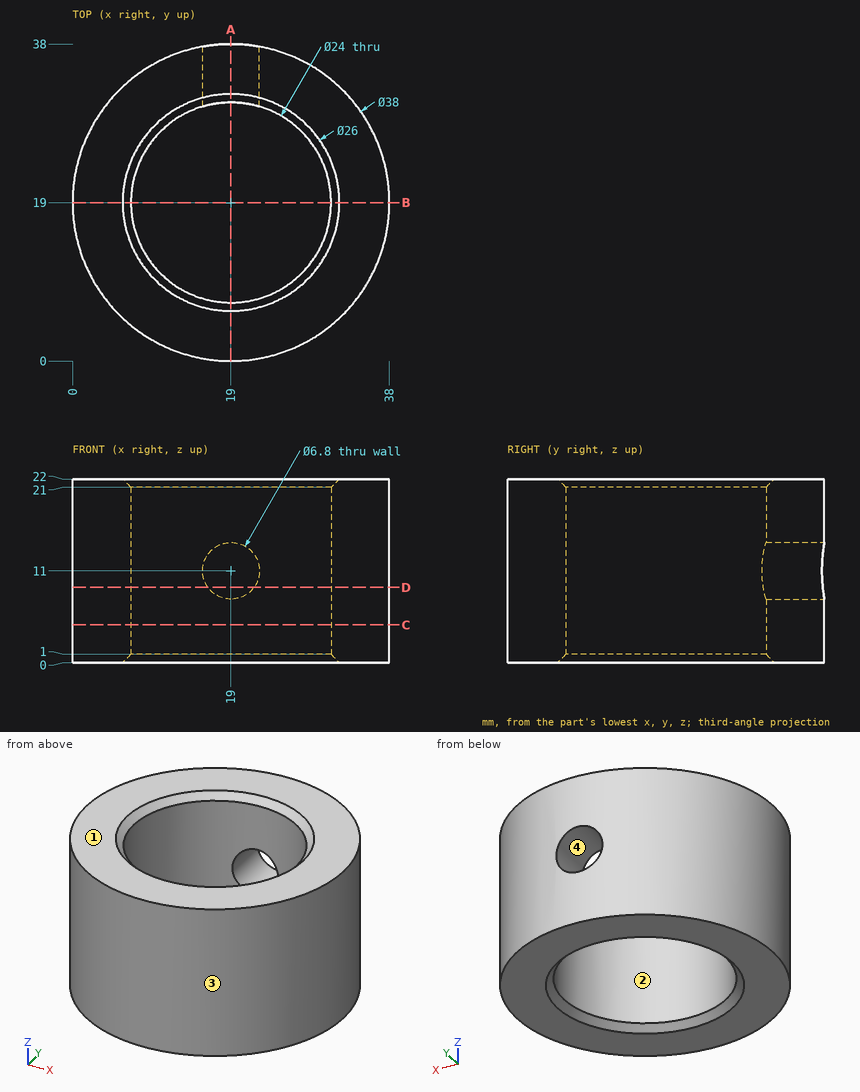
Job drawing, mm, ordinate dimensions from the low corner. One solid piece. Give positions to 0.01 mm unless a question says otherwise; leave off trailing zeros. Order: outer loops, then holes, each group sorted by start corner. A loop starts at its lowest first (then second) coordinate and runs counter-clockwise, first axis right, second up. Notation, with made-up numbers: (13.5, 34.25) - (27.5, 34.25) arc R15 ccw to (27.5, 39.25) - close; hole circle Ø8 at (10, -31.75). An arc over 180 degrees is marked (long way). Answer in a Markdown table with one row per item.
1. Flat gauge pins, fed straight in: pin 1 (1 mm diameter, centred on x = 5, z = 14.5, fed in from -Y); pin 2 (4 mm diameter, centred on x = 34, z = 12.5, fed in from +Y); pin 3 (12 mm diameter, centred on x = 25, y = 13, fed in from -Z); pin 4 (5 mm diameter, centred on x = 7.5, z = 10.5, fed in from +Y). Where does each tip first touch, or does it go through?
Data:
| item | result |
|---|---|
| pin 1 | stops at y = 5.63 |
| pin 2 | stops at y = 32.86 |
| pin 3 | stops at z = 0 |
| pin 4 | stops at y = 35.73 |
2. Saw through at B-B, the plane y = 19. Give the cut face in (x, z), plus the area to 3 significant figures.
Data:
| item | result |
|---|---|
| outline | (0, 0) - (6, 0) - (7, 1) - (7, 21) - (6, 22) - (0, 22) - close; (31, 1) - (32, 0) - (38, 0) - (38, 22) - (32, 22) - (31, 21) - close |
| area | 306 mm² |
3. Saw through at A-A, the plane x = 19. Give the cut face in (y, z).
Data:
| item | result |
|---|---|
| outline | (0, 0) - (6, 0) - (7, 1) - (7, 21) - (6, 22) - (0, 22) - close; (31, 1) - (32, 0) - (38, 0) - (38, 7.6) - (31, 7.6) - close; (31, 14.4) - (38, 14.4) - (38, 22) - (32, 22) - (31, 21) - close |
4. Pull direction X, two halves, no side cores. Call the marked faces 1, 2, 3 and 4: pulls with the +X half, pulls with the -X half, needs draft (parallel to the pull), parting line crosses it, or undercut.
Data:
| item | result |
|---|---|
| face 1 | needs draft |
| face 2 | undercut |
| face 3 | parting line crosses it |
| face 4 | undercut |
5. Probe probe 1 along Y at (x, z) = (20.5, 17); probe 2 along Y at (x, z) = (25.5, 20); probe 3 along X at (y, z) = (23.5, 2.5). List the from-to ranges inside material, lowest first. Write a range as [from, to].
Data:
| item | result |
|---|---|
| probe 1 | y = [0.06, 7.09], [30.91, 37.94] |
| probe 2 | y = [1.15, 8.91], [29.09, 36.85] |
| probe 3 | x = [0.54, 7.88], [30.12, 37.46] |
6. Saw through at D-D, the plane z = 9. Give the cut face in (x, y), plus the area to 3 significant figures.
Data:
| item | result |
|---|---|
| outline | (16.25, 30.68) - (16.25, 37.8) arc R19 ccw (long way) to (21.75, 37.8) - (21.75, 30.68) arc R12 cw (long way) to start |
| area | 643 mm² |
7. Saw through at C-C, the plane z = 4.5. Give the cut face in (x, y), plus the area to 3 significant figures.
Data:
| item | result |
|---|---|
| outline | circle Ø38 at (19, 19); hole circle Ø24 at (19, 19) |
| area | 682 mm² |
